from build123d import *

# Parameters (mm, degrees)
SKETCH4_R           = 63
SKETCH4_R_2         = 32.5
BOSS_EXTRUDE1_DEPTH = 15.5
SKETCH5_R           = 63
SKETCH5_R_2         = 60
BOSS_EXTRUDE2_DEPTH = 22
SKETCH7_W           = 25
SKETCH7_H           = 24.247693635
CUT_EXTRUDE1_DEPTH  = 5


with BuildPart() as part:
    # Sketch4 → Boss-Extrude1 (new body)
    with BuildSketch(Plane(origin=(0, 0, 0), x_dir=(1, 0, 0), z_dir=(0, 1, 0))):
        Circle(SKETCH4_R)
        Circle(SKETCH4_R_2, mode=Mode.SUBTRACT)
    extrude(amount=BOSS_EXTRUDE1_DEPTH)

    # Sketch5 → Boss-Extrude2 (add)
    with BuildSketch(Plane(origin=(0, 15.5, 0), x_dir=(1, 0, 0), z_dir=(0, 1, 0))):
        Circle(SKETCH5_R)
        Circle(SKETCH5_R_2, mode=Mode.SUBTRACT)
    extrude(amount=BOSS_EXTRUDE2_DEPTH)

    # Sketch7 → Cut-Extrude1 (cut)
    with BuildSketch(Plane(origin=(0, 15.5, 0), x_dir=(1, 0, 0), z_dir=(0, 1, 0))):
        with Locations((32.454830069, 1.71289381)):
            Rectangle(SKETCH7_W, SKETCH7_H)
    extrude(amount=-CUT_EXTRUDE1_DEPTH, mode=Mode.SUBTRACT)


solid = part.part
Build history of the part. All positions in model axes, mm. A direction names the side the tool comes from. Round coordinates to 2 decimals unless told otherwise and drop trailing zeros. Write each loop counter-clockwise with the first axis right and the second up, starting at its lowest first coordinate (ties: lowest second). Pieces come first, ordered by that corner, then holes. Notation, with made-up numbers: (-37, -5.75) -> (-24, -5.75) arc R29 ccw to (-24, 15.25) -> close; hole circle Ø1 at (46, -8.75). An arc over 180 degrees is marked (long way). Write item = value, one per line.
(1) Tool access for faces 1 (the face through (27, 0, 27)), 2 (the face through (37, 13, -13.837)): list every direction of +Z, -Z, +X, -X, +Y, -Y with a clear straight run to the whole face (end or side of a thin tool).
Answer:
face_1 = +Z, -Z, +X, -X, -Y
face_2 = +Y
(2) Probe L1, parallel to X at y = 32, z = 0; L2, parallel to X at y = 11.75, z = 0. List the from-to ranges inside material, lowest first.
Answer:
L1 = -63 to -60, 60 to 63
L2 = -63 to -32.5, 44.95 to 63
(3) Band-saw the part on A-A (x = 0). Give the cut face in (y, z).
Answer:
outline = (0, -63) -> (37.5, -63) -> (37.5, -60) -> (15.5, -60) -> (15.5, -32.5) -> (0, -32.5) -> close; (0, 32.5) -> (15.5, 32.5) -> (15.5, 60) -> (37.5, 60) -> (37.5, 63) -> (0, 63) -> close
(4) Flat gauge pins, fed straight in: pin 1 (3 mm diameter, centred on x = 31, z = -37.5, fed in from +Y); pin 2 (12.5 mm diameter, centred on x = 37.5, z = -2, fed in from +Y); pin 3 (2.5 mm diameter, centred on y = 12.5, z = -7, fed in from -X). Where does each tip first touch, or does it go through?
Answer:
pin_1 = 15.5
pin_2 = 10.5
pin_3 = -62.74
(5) Two-plate mould, pull along Z, no slides. Class faces 3 (the face through (-8.201, 18.488, -62.464)), 4 (the face through (56, 37.5, 23)), 5 (the face through (-59.94, 26.35, -2.64)): pulls with the +Z half, pulls with the -Z half, needs draft (parallel to the pull), parting line crosses it, or undercut.
Answer:
face_3 = parting line crosses it
face_4 = needs draft
face_5 = undercut
(6) Band-saw the part on D-D (x = 46.5). Give the cut face in (y, z).
Answer:
outline = (0, -42.51) -> (37.5, -42.51) -> (37.5, -37.92) -> (15.5, -37.92) -> (15.5, 37.92) -> (37.5, 37.92) -> (37.5, 42.51) -> (0, 42.51) -> close
(7) Band-saw the part on B-B (z = 0). Give the cut face in (x, y), then the cut area to 3 significant figures.
Answer:
outline = (-63, 0) -> (-32.5, 0) -> (-32.5, 15.5) -> (-60, 15.5) -> (-60, 37.5) -> (-63, 37.5) -> close; (32.5, 0) -> (63, 0) -> (63, 37.5) -> (60, 37.5) -> (60, 15.5) -> (44.95, 15.5) -> (44.95, 10.5) -> (32.5, 10.5) -> close
area = 1,020 mm2
(8) Band-saw the part on C-C (y = 23). Give the cut face in (x, z), then the cut area to 3 significant figures.
Answer:
outline = circle Ø126 at (0, 0); hole circle Ø120 at (0, 0)
area = 1,160 mm2
